from build123d import *

# Parameters (mm, degrees)
F0_W     = 118.813
F0_H     = 20
F1_DEPTH = 4
F2_T     = 2.5
F3_R     = 3


# Not quite as in the source:
# - a shell that OpenCascade refuses in one call is made with other operations: the cavity is built on its own and cut out


with BuildPart() as f1:
    # F0 (on Front) → F1 (new body)
    with BuildSketch(Plane.XZ):
        Rectangle(F0_W, F0_H)
        with BuildLine():
            Line((-33.4065, -7.5), (-53.4065, -7.5))
            ThreePointArc((-53.4065, -7.5), (-55.9065, -5), (-53.4065, -2.5))
            Line((-53.4065, -2.5), (-33.4065, -2.5))
            ThreePointArc((-33.4065, -2.5), (-30.9065, -5), (-33.4065, -7.5))
        make_face(mode=Mode.SUBTRACT)
        with BuildLine():
            Line((53.4065, -7.5), (33.4065, -7.5))
            ThreePointArc((33.4065, -7.5), (30.9065, -5), (33.4065, -2.5))
            Line((33.4065, -2.5), (53.4065, -2.5))
            ThreePointArc((53.4065, -2.5), (55.9065, -5), (53.4065, -7.5))
        make_face(mode=Mode.SUBTRACT)
        with BuildLine():
            Line((-33.4065, 1.9), (-53.4065, 1.9))
            ThreePointArc((-53.4065, 1.9), (-56.5065, 5), (-53.4065, 8.1))
            Line((-53.4065, 8.1), (-33.4065, 8.1))
            ThreePointArc((-33.4065, 8.1), (-30.3065, 5), (-33.4065, 1.9))
        make_face(mode=Mode.SUBTRACT)
        with BuildLine():
            Line((53.4065, 1.9), (33.4065, 1.9))
            ThreePointArc((33.4065, 1.9), (30.3065, 5), (33.4065, 8.1))
            Line((33.4065, 8.1), (53.4065, 8.1))
            ThreePointArc((53.4065, 8.1), (56.5065, 5), (53.4065, 1.9))
        make_face(mode=Mode.SUBTRACT)
    extrude(amount=F1_DEPTH)

    # F2: shell of thickness 2.5, made by hand


with BuildPart() as f2_core1:
    # F2_t2: copy of F1
    add(f1.part)

    # the walls: a layer under each face that stays
    f2_faces = [f2_core1.faces().sort_by_distance(p)[0] for p in [
        (59.4065, -2, 0),
        (0, -2, 10),
        (-59.4065, -2, 0),
        (0, -2, -10),
        (-43.4065, -2, -7.5),
        (-55.9065, -2, -5),
        (-43.4065, -2, -2.5),
        (-30.9065, -2, -5),
        (43.4065, -2, -7.5),
        (30.9065, -2, -5),
        (43.4065, -2, -2.5),
        (55.9065, -2, -5),
        (-43.4065, -2, 8.1),
        (-30.3065, -2, 5),
        (-43.4065, -2, 1.9),
        (-56.5065, -2, 5),
        (43.4065, -2, 1.9),
        (30.3065, -2, 5),
        (43.4065, -2, 8.1),
        (56.5065, -2, 5),
    ]]
    thicken(f2_faces, amount=-F2_T, mode=Mode.SUBTRACT)


with BuildPart() as f1_1:
    add(f1.part)

    # what is left inside the walls is the cavity
    f2_cavity = [f2_core1.part.solids().sort_by_distance(p)[0] for p in [
        (56.105376, -2.666667, -0.761286),
        (0, -0.025, -2.5),
        (-56.105376, -2.666667, -0.761286),
    ]]
    add(f2_cavity, mode=Mode.SUBTRACT)

    # F3
    f3_edges = [f1_1.edges().sort_by_distance(p)[0] for p in [
        (59.4065, -2, -10),
        (59.4065, -2, 10),
        (-59.4065, -2, -10),
        (-59.4065, -2, 10),
    ]]
    fillet(f3_edges, radius=F3_R)


solid = f1_1.part
Verification items for the finished model (mm, model axes). A direction names the side the tool comes from. Give positions to 0.01 mm unless a question says otherwise; leave off trailing zeros. Loops run counter-clockwise (first coordinate to the right, second up) from the corner with the lowest first, then second, coordinate; pieces in that order, holes last. Notation, with made-up numbers: (-31, 68.5) - (13, 68.5) arc R16 cw to (13, 90.5) - close; hole circle Ø7 at (-1, 89). An arc over 180 degrees is marked (long way). Write item = value, one per line. Start each with the question number.
Q1. Cross-section at D-D, the plane z = -5. Enter the section's corners in (x, y).
Q2. Cross-section at A-A, the plane x = 45.5. Enter the section's corners in (y, z).
Q3. Tool access check on faces 5 (the face through (0, 0, -8)), 6 (the face through (-56.506, -1.972, 4.932)). Record the directions out of +Z, -Z, +X, -X, +Y, -Y that give a thin tool (end or side, any length) a straight path to the whole face; none if there is none.
Q4. Cross-section at C-C, the plane x = -9. Enter the section's corners in (y, z).
Q5. Mould release check, pull along Z, two halves, no side actions. Record for faces 1 (the face through (-30.907, -1.972, -4.945)), 2 (the face through (28.68, -1.97, -3.37)), 3 (the face through (-58.55, -2.03, -9.1)), 4 (the face through (59.406, -2, 0)): released by +Z, released by -Z, zero draft, split by the parting line, or undercut.
Q6. Cross-section at B-B, the plane z = 5. Enter the section's corners in (x, y).
Q7. Thickness scan on line 1 (X direction, y = -1.5, z = 0); line 2 (Z direction, x = -50, y = -1.55); line 3 (X direction, y = -1.7, z = -5). Record the ranges inside material, lowest first.
Answer key:
q1.outline = (-59.41, -4) - (-55.91, -4) - (-55.91, 0) - (-59.41, 0) - close; (-30.91, -4) - (-28.41, -4) - (-28.41, 0) - (-30.91, 0) - close; (28.41, -4) - (30.91, -4) - (30.91, 0) - (28.41, 0) - close; (55.91, -4) - (59.41, -4) - (59.41, 0) - (55.91, 0) - close
q2.outline = (-4, -10) - (0, -10) - (0, -7.5) - (-4, -7.5) - close; (-4, -2.5) - (0, -2.5) - (0, 1.9) - (-4, 1.9) - close; (-4, 8.1) - (0, 8.1) - (0, 10) - (-4, 10) - close
q3.face_5 = +Z, -Z, +X, -X, +Y
q3.face_6 = +Y, -Y
q4.outline = (-4, -10) - (0, -10) - (0, -7.5) - (-4, -7.5) - close; (-4, 7.5) - (0, 7.5) - (0, 10) - (-4, 10) - close
q5.face_1 = undercut
q5.face_2 = undercut
q5.face_3 = released by -Z
q5.face_4 = zero draft
q6.outline = (-59.41, -4) - (-56.51, -4) - (-56.51, 0) - (-59.41, 0) - close; (-30.31, -4) - (-27.81, -4) - (-27.81, 0) - (-30.31, 0) - close; (27.81, -4) - (30.31, -4) - (30.31, 0) - (27.81, 0) - close; (56.51, -4) - (59.41, -4) - (59.41, 0) - (56.51, 0) - close
q7.line_1 = -59.41 to -56.91, -55.93 to -30.88, 30.88 to 55.93, 56.91 to 59.41
q7.line_2 = -10 to -7.5, -2.5 to 1.9, 8.1 to 10
q7.line_3 = -59.41 to -55.91, -30.91 to -28.41, 28.41 to 30.91, 55.91 to 59.41
